```python
from build123d import *
from build123d.topology import SkipClean

# Parameters (mm, degrees)
SKETCH1_R               = 40
BOSS_EXTRUDE1_DEPTH     = 100
CUT_EXTRUDE1_START      = -10
CUT_EXTRUDE1_DEPTH      = 180
CUT_EXTRUDE2_DEPTH      = 208.846096908
CUT_EXTRUDE2_DEPTH_BACK = 208.846096908
SKETCH3_R               = 2.5
BOSS_EXTRUDE2_START     = -165
SKETCH4_R               = 41
SKETCH4_R_2             = 40
BOSS_EXTRUDE2_DEPTH     = 130
SCALE1_SCALE            = 1.1


with BuildPart() as part:
    # Sketch1 → Boss-Extrude1 (new, symmetric)
    with BuildSketch(Plane.XY):
        Circle(SKETCH1_R)
        with BuildLine():
            Line((29.580398915, 5), (-29.580398915, 5))
            ThreePointArc((-29.580398915, 5), (0, 30), (29.580398915, 5))
        make_face(mode=Mode.SUBTRACT)
        with BuildLine():
            Line((29.580398915, -5), (-29.580398915, -5))
            ThreePointArc((-29.580398915, -5), (0, -30), (29.580398915, -5))
        make_face(mode=Mode.SUBTRACT)
    extrude(amount=BOSS_EXTRUDE1_DEPTH, both=True)

    # Sketch2 → Cut-Extrude1 (cut)
    with BuildSketch(Plane.XY.offset(100).offset(CUT_EXTRUDE1_START)):
        with BuildLine():
            Line((-29.580398915, 5), (29.580398915, 5))
            ThreePointArc((29.580398915, 5), (30, 0), (29.580398915, -5))
            Line((29.580398915, -5), (-29.580398915, -5))
            ThreePointArc((-29.580398915, -5), (-30, 0), (-29.580398915, 5))
        make_face()
    extrude(amount=-CUT_EXTRUDE1_DEPTH, mode=Mode.SUBTRACT)

    # Sketch3 → Cut-Extrude2 (cut, two sides: drawn at the far end of the back side and taken through both)
    with SkipClean():  # the faces are left unmerged after this step: merging them gives an invalid solid
        with BuildSketch(Plane.XY.offset(100).offset(-CUT_EXTRUDE2_DEPTH_BACK)):
            Circle(SKETCH3_R)
        extrude(amount=CUT_EXTRUDE2_DEPTH + CUT_EXTRUDE2_DEPTH_BACK, mode=Mode.SUBTRACT)

    # Sketch4 → Boss-Extrude2 (add)
    with SkipClean():  # the faces are left unmerged after this step: merging them gives an invalid solid
        with BuildSketch(Plane(origin=(0, 0, -100), x_dir=(-1, 0, 0), z_dir=(0, 0, -1)).offset(BOSS_EXTRUDE2_START)):
            Circle(SKETCH4_R)
            Circle(SKETCH4_R_2, mode=Mode.SUBTRACT)
        extrude(amount=BOSS_EXTRUDE2_DEPTH)


with BuildPart() as part_1:
    # Scale1: scaled about (0, 0, 0)
    add(part.part.scale(SCALE1_SCALE))


solid = part_1.part
```
The model under review builds one solid part; all positions refer to its coordinate system, in mm. A direction names the side the tool comes from. Coordinates: 2 decimals unless noted, no trailing zeros. Write each loop counter-clockwise with the first axis right and the second up, starting at its lowest first coordinate (ties: lowest second). Pieces come first, ordered by that corner, then holes. Notation, with made-up numbers: (85, 12.25) - (96, 12.25) arc R20 cw to (96, 29.25) - close; hole circle Ø11 at (38, 12). An arc over 180 degrees is marked (long way). Answer in a Markdown table with one row per item. Add a question column.
Q1. Draft analysis for pull direction Z (two halves, no side actions). For faces 4 (the face through (-9.8, -43.2, -71.5)), 5 (the face through (-9.8, -43.2, 71.5)), 6 (the face through (0, 4, 99)), 7 (the face through (-0.596, -2.685, 104.423)), state which applies: +Z half, -Z half, draft (parallel to the pull), parting line (faces both ways), or undercut.
Q2. Consider section B-B on x = 0. Give the number of separate pieces and of enclosed holes in the cut face, then the cut area to 3 significant figures.
Q3. Consider section C-C on x = -22.5. Give the boundary of the cut face in (y, z), then the cut area to 3 significant figures.
Q4. Clearance check with flat-ended pins moving along their axes: pin 1 (9 mm diameter, centred on x = 0, y = 0, fed in from +Z); pin 2 (3 mm diameter, centred on x = -28, z = -26, fed in from -Y); pin 3 (9 mm diameter, centred on x = -7, z = -104.5, fed in from +Y); pin 4 (3 mm diameter, centred on x = -22, z = -81, fed in from -Y). State where each tip first meets the part, or that it passes through.
Q5. To check wall thickness, follow line 1 along Y through (x, z) = (0, -101); line 2 along Z through (x, y) = (25.5, -2.5); line 3 along Y through (x, z) = (-28, 37). State the ranges of each line that lie inside material, in increasing order. Write a range as from..to.
Q6. Consider section A-A on y = 0. Give the boundary of the cut face in (x, z), then the cut area to 3 significant figures.
Q7. Consider section D-D on z = -43. Give the boundary of the cut face in (x, y), then the cut area to 3 significant figures.
Q8. For faces 1 (the face through (-9.538, -42.954, 91.02)), 2 (the face through (-9.538, -42.954, -90.48)), 3 (the face through (0, -5.5, 105)), list the 3-axis set-ups (+Z, -Z, +X, -X, +Y, -Y) from which the entire face can be reached by the end or side of a thin tool; tool diameter is ignored.
Answers below:
| question | item | result |
|---|---|---|
| 1 | face 4 | -Z half |
| 1 | face 5 | +Z half |
| 1 | face 6 | undercut |
| 1 | face 7 | draft |
| 2 | separate pieces | 6 |
| 2 | enclosed holes | 0 |
| 2 | area | 5,280 mm² |
| 3 | outline | (-39.09, -71.5) - (-37.81, -71.5) - (-37.81, -110) - (-24.14, -110) - (-24.14, 110) - (-37.81, 110) - (-37.81, 71.5) - (-39.09, 71.5) - close; (-5.5, -110) - (5.5, -110) - (5.5, -99) - (-5.5, -99) - close; (-5.5, 99) - (5.5, 99) - (5.5, 110) - (-5.5, 110) - close; (24.14, -110) - (37.81, -110) - (37.81, -71.5) - (39.09, -71.5) - (39.09, 71.5) - (37.81, 71.5) - (37.81, 110) - (24.14, 110) - close |
| 3 | area | 6,620 mm² |
| 4 | pin 1 | z = 110 |
| 4 | pin 2 | y = -36.49 |
| 4 | pin 3 | y = 43.93 |
| 4 | pin 4 | y = -38.93 |
| 5 | line 1 | -44..-33, -5.5..-2.75, 2.75..5.5, 33..44 |
| 5 | line 2 | -110..-99, 99..110 |
| 5 | line 3 | -35.36..-17.46, 17.46..35.36 |
| 6 | outline | (-45.1, -71.5) - (-44, -71.5) - (-44, -110) - (-2.75, -110) - (-2.75, -99) - (-33, -99) - (-33, 99) - (-2.75, 99) - (-2.75, 110) - (-44, 110) - (-44, 71.5) - (-45.1, 71.5) - close; (2.75, -110) - (44, -110) - (44, -71.5) - (45.1, -71.5) - (45.1, 71.5) - (44, 71.5) - (44, 110) - (2.75, 110) - (2.75, 99) - (33, 99) - (33, -99) - (2.75, -99) - close |
| 6 | area | 6,490 mm² |
| 7 | outline | circle Ø90.2 at (0, 0); hole circle Ø66 at (0, 0) |
| 7 | area | 2,970 mm² |
| 8 | face 1 | +Z |
| 8 | face 2 | -Z |
| 8 | face 3 | +Z, -Z |
